The model under review builds one solid part; all positions refer to its coordinate system, in mm. A direction names the side the tool comes from. Give positions to 0.01 mm unless a question says otherwise; leave off trailing zeros. Loops run counter-clockwise (first coordinate to the right, second up) from the corner with the lowest first, then second, coordinate; pieces in that order, holes last. Notation, with made-up numbers: (46.5, -13.5) -> (91.5, -13.5) arc R27 cw to (91.5, 6.5) -> close; hole circle Ø11 at (18, 13). An arc over 180 degrees is marked (long way). Write each question's results on one line, items separated by ' | '. Start each with the question number.
Q1. We need section A-A (x = 376). Write out the cut boundary in (y, z), plus the area to 3 significant figures.
Q2. Mouldability with a two-part tool opening along X and no side actions: class faces 1 (the face through (200, 0.794, 7)), 2 (the face through (259.866, 11.062, 0.402)), 3 (the face through (0, 13.4, 0.2)) as released by +X, released by -X, zero draft, split by the parting line, or undercut.
Q3. Insertion check: pin 1 Ø5 at (x, y) = (153.5, 10) entering from +Z; pin 2 Ø1.9 at (x, z) = (254, 7.94) entering from -Y. Each pin has a flat end and moves straight along its axis. Give the tip position at first contact, or say it passes through.
Q4. Wall thickness on L1, parallel to Y at x = 295, z = 4; L2, parallel to Z at x = 254, y = 26.4 (3 decimals); L3, parallel to Y at x = 254, z = 0.4: over which ranges is each line inside the solid? List them lowest first. Write a range as [from, to].
Q5. Machinability: for faces 4 (the face through (200, 14, 0.794)), 5 (the face through (406.4, 13.4, 0.2)), which of the approach directions +Z, -Z, +X, -X, +Y, -Y give a long, thin tool a straight path to every point of the face, cutting with its end or side? Answer none if there is none.
from build123d import *

# Parameters (mm, degrees)
F0_W     = 406.4
F0_H     = 26.9875
F1_DEPTH = 0.79375
F2_W     = 406.4
F2_H     = 0.79375
F3_DEPTH = 12.7
F4_R     = 1.5875
F5_DEPTH = 26.9885
F6_R     = 6.35
F6_R_2   = 2.38125
F7_DEPTH = 25.4


with BuildPart() as f1:
    # F0 (on Top) → F1 (new body)
    with BuildSketch(Plane.XY):
        with Locations((203.2, 13.49375)):
            Rectangle(F0_W, F0_H)
    extrude(amount=F1_DEPTH)

    # F2 (on face) → F3 (join)
    with BuildSketch(Plane.XY.offset(0.79375)):
        with Locations((203.2, 26.590625)):
            Rectangle(F2_W, F2_H)
        with Locations((203.2, 0.396875)):
            Rectangle(F2_W, F2_H)
    extrude(amount=F3_DEPTH)

    # F4 (on face) → F5 (cut, through all)
    with BuildSketch(Plane.XZ):
        with Locations((311.15, 7.9375)):
            Circle(F4_R)
        with Locations((254, 7.9375)):
            Circle(F4_R)
        with Locations((40.48125, 7.9375)):
            Circle(F4_R)
        with Locations((9.525, 7.9375)):
            Circle(F4_R)
    extrude(amount=-F5_DEPTH, mode=Mode.SUBTRACT)

    # F6 (on face) → F7 (cut)
    with BuildSketch(Plane.XY.offset(0.79375)):
        with Locations((254, 13.49375)):
            Circle(F6_R)
        with Locations((361.95, 13.49375)):
            Circle(F6_R_2)
    extrude(amount=-F7_DEPTH, mode=Mode.SUBTRACT)


solid = f1.part
Output:
1) outline: (0, 0) -> (26.99, 0) -> (26.99, 13.49) -> (26.19, 13.49) -> (26.19, 0.79) -> (0.79, 0.79) -> (0.79, 13.49) -> (0, 13.49) -> close | area: 41.6 mm2
2) face 1: zero draft | face 2: undercut | face 3: released by -X
3) pin 1: z = 0.79 | pin 2: through
4) L1: [0, 0.79], [26.19, 26.99] | L2: [0, 6.35], [9.525, 13.494] | L3: [0, 7.14], [19.84, 26.99]
5) face 4: +Z, +X, -X | face 5: +Z, -Z, +X, +Y, -Y
